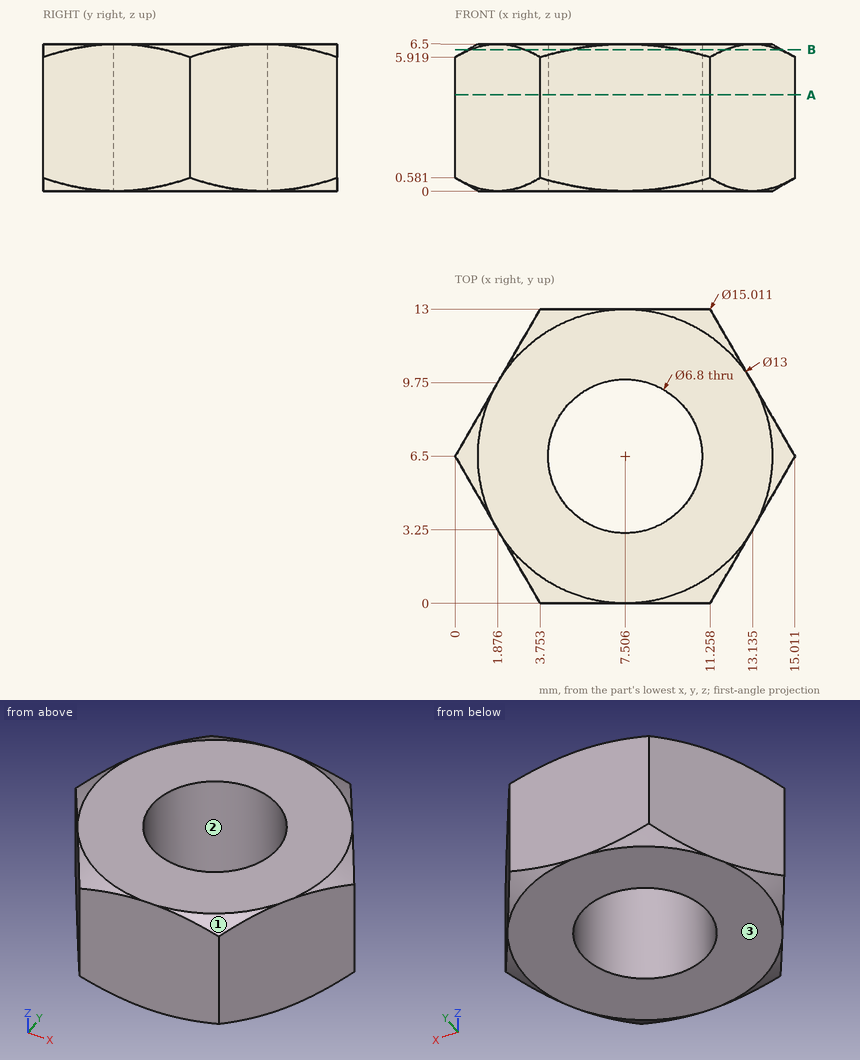
Print and shaded views of the part. All mm, measured from the part's lowest x, y and z. Round coordinates to 2 decimals unless told otherwise and drop trailing zeros. Order: outer loops, then holes, each group sorted by start corner. A loop starts at its lowest first (then second) coordinate and runs counter-clockwise, first axis right, second up.
Q1. Wall check: L1, parallel to Y at x = 10, z = 6; L2, parallel to X at y = 3.5, z = 5.75 (1 decimal); L3, parallel to X at y = 6.25, z = 5.25 (1 decimal). Give the ranges that are in metal, low to high.
Q2. Slice it at A-A (z = 4.25). Write the cut outline in (x, y) (1 decimal).
Q3. Drop flat-ended pins along their axis: pin 1 (6 mm diameter, centred on x = 7.51, y = 6.5, fed in from -Z); pin 2 (1.5 mm diameter, centred on y = 9.5, z = 4, fed in from +X). Give the stop position or say it passes through.
Q4. Two-plate mould, pull along X, no slides. Class the marked faces 1, 2 and 3: pulls with the +X half, pulls with the -X half, needs draft (parallel to the pull), parting line crosses it, or undercut.
Q5. Slice it at B-B (z = 6.25). Write the cut outline in (x, y) (1 decimal).
Results below:
1. L1: y = 0 to 4.19, 8.81 to 13
1. L2: x = 1.7 to 5.9, 9.1 to 13.3
1. L3: x = 0.1 to 4.1, 10.9 to 14.9
2. outline: (0, 6.5) - (3.8, 0) - (11.3, 0) - (15, 6.5) - (11.3, 13) - (3.8, 13) - close; hole circle Ø6.8 at (7.5, 6.5)
3. pin 1: passes through
3. pin 2: stops at x = 13.71
4. face 1: pulls with the +X half
4. face 2: undercut
4. face 3: needs draft
5. outline: (0.7, 5.3) - (3.1, 1.2) arc R6.9 ccw to (5.1, 0) - (9.9, 0) arc R6.9 ccw to (11.9, 1.2) - (14.3, 5.3) arc R6.9 ccw to (14.3, 7.7) - (11.9, 11.8) arc R6.9 ccw to (9.9, 13) - (5.1, 13) arc R6.9 ccw to (3.1, 11.8) - (0.7, 7.7) arc R6.9 ccw to start; hole circle Ø6.8 at (7.5, 6.5)
